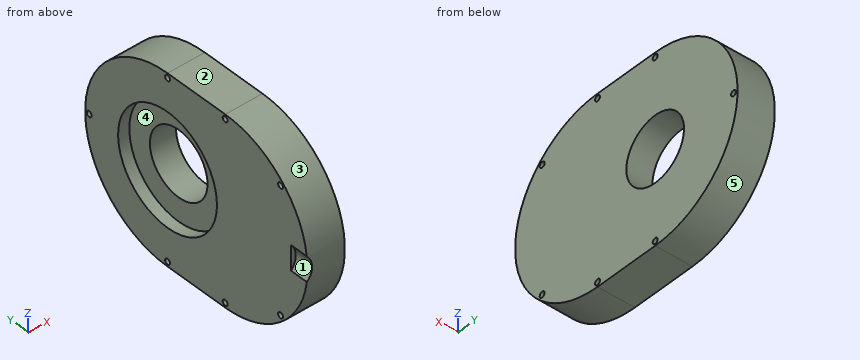
from build123d import *

# Parameters (mm, degrees)
CROQUIS1_R              = 17.5
SALIENTE_EXTRUIR1_DEPTH = 20
CROQUIS2_R              = 30
CORTAR_EXTRUIR1_DEPTH   = 6
CROQUIS3_R              = 10
CORTAR_EXTRUIR2_DEPTH   = 10
CROQUIS4_R              = 1.5
CORTAR_EXTRUIR3_DEPTH   = 101.623059057


with BuildPart() as part:
    # Croquis1 → Saliente-Extruir1 (new body)
    with BuildSketch(Plane(origin=(0, 0, 0), x_dir=(0, 0, -1), z_dir=(1, 0, 0))):
        with BuildLine():
            Line((-50, 35), (-50, 0))
            ThreePointArc((-50, 0), (0, -50), (50, 0))
            Line((50, 0), (50, 35))
            ThreePointArc((50, 35), (0, 85), (-50, 35))
        make_face()
        with Locations((0, 35)):
            Circle(CROQUIS1_R, mode=Mode.SUBTRACT)
    extrude(amount=SALIENTE_EXTRUIR1_DEPTH)

    # Croquis2 → Cortar-Extruir1 (cut)
    with BuildSketch(Plane(origin=(0, 0, 0), x_dir=(0, 0, -1), z_dir=(1, 0, 0))):
        with Locations((0, 35)):
            Circle(CROQUIS2_R)
    extrude(amount=CORTAR_EXTRUIR1_DEPTH, mode=Mode.SUBTRACT)

    # Croquis3 → Cortar-Extruir2 (cut)
    with BuildSketch(Plane(origin=(0, -50, 0), x_dir=(1, 0, 0), z_dir=(0, 1, 0))):
        with Locations((-7.5, 0)):
            Circle(CROQUIS3_R)
    extrude(amount=CORTAR_EXTRUIR2_DEPTH, mode=Mode.SUBTRACT)

    # Croquis4 → Cortar-Extruir3 (cut, through all)
    with BuildSketch(Plane.ZY):
        with Locations((0, 82.5)):
            Circle(CROQUIS4_R)
        with Locations((47.5, 35)):
            Circle(CROQUIS4_R)
        with Locations((-47.5, 35)):
            Circle(CROQUIS4_R)
        with Locations((-47.5, 0)):
            Circle(CROQUIS4_R)
        with Locations((47.5, 0)):
            Circle(CROQUIS4_R)
        with Locations((33.587572106, -33.587572106)):
            Circle(CROQUIS4_R)
        with Locations((-33.587572106, -33.587572106)):
            Circle(CROQUIS4_R)
    extrude(amount=-CORTAR_EXTRUIR3_DEPTH, mode=Mode.SUBTRACT)


solid = part.part
Model file for the job. Use its own axes, mm. Face numbers are marked on the shaded views. A direction names the side the tool comes from. Round coordinates to 2 decimals unless told otherwise and drop trailing zeros. Order: outer loops, then holes, each group sorted by start corner. A loop starts at its lowest first (then second) coordinate and runs counter-clockwise, first axis right, second up. Notation, with made-up numbers: M 76.5,76.25 L 122.5,76.25 A32 cw 122.5,105.25 Z; hole C 39,50.5 d10. An arc over 180 degrees is marked long. Write each question's results on one line, items separated by ' | '. Start each with the question number.
(1) Saw through at A-A, the plane y = 82.5. Give the cut face in (x, z).
(2) Two-plate mould, pull along Z, no slides. Class the marked faces 1, 2 and 3: pulls with the +Z half, pulls with the -Z half, needs draft (parallel to the pull), parting line crosses it, or undercut.
(3) Drop flat-ended pins along their axis: pin 1 (1.5 mm diameter, centred on x = 14.5, y = -25, fed in from -Z); pin 2 (1.5 mm diameter, centred on x = 4.5, y = 69.5, fed in from +Z); pin 3 (5 mm diameter, centred on x = 8, z = 24, fed in from +Y). Give the stop position or say it passes through.
(4) Saw through at C-C, the plane z = -14. Give the cut face in (x, y), then the cut area to 3 significant figures.
(5) Saw through at D-D, the plane z = 47.5. Give the cut face in (x, y).
(6) Which spindle directions (+Z, -Z, +X, -X, +Y, -Y) get a long thin tool onto all of the face, cutting with end or side? Do the marked faces 4 and 5. Say none if no direction does.
(7) Saw through at B-B, the plane x = 17.25. State how many separate pieces and enclosed holes the cut face has, then the cut area to 3 significant figures.
(8) Probe probe 1 along Y at (x, z) = (7.75, 0); probe 2 along Z at (x, y) = (13, 25); probe 3 along Y at (x, z) = (19, -33.5). List the from-to ranges inside material, lowest first. Write a range as from..to.
Established:
1) outline: M 0,-15.61 L 20,-15.61 L 20,-1.5 L 0,-1.5 Z; M 0,1.5 L 20,1.5 L 20,15.61 L 0,15.61 Z
2) face 1: undercut | face 2: pulls with the +Z half | face 3: parting line crosses it
3) pin 1: stops at z = -43.73 | pin 2: stops at z = 36.89 | pin 3: stops at y = 80.14
4) outline: M 0,-48 L 20,-48 L 20,24.5 L 6,24.5 L 6,8.47 L 0,8.47 Z; M 0,61.53 L 6,61.53 L 6,45.5 L 20,45.5 L 20,83 L 0,83 Z | area: 2,010 mm^2
5) outline: M 0,-15.61 L 20,-15.61 L 20,-1.5 L 0,-1.5 Z; M 0,1.5 L 20,1.5 L 20,33.5 L 0,33.5 Z; M 0,36.5 L 20,36.5 L 20,50.61 L 0,50.61 Z
6) face 4: -X | face 5: +X, -X, +Y
7) separate pieces: 1 | enclosed holes: 8 | area: 10,300 mm^2
8) probe 1: y = -50..17.5, 52.5..81, 84..85 | probe 2: z = -50..-14.36, 14.36..50 | probe 3: y = -37.12..-35.09, -32.09..72.12
